```python
from build123d import *

# Parameters (mm, degrees)
F0_W     = 32
F0_H     = 10
F0_R     = 1.6
F1_DEPTH = 3.5
F2_R     = 4.99999
F3_R     = 1


# Not quite as in the source:
# - a fillet or chamfer is up to 0.001 mm smaller than in the source, because OpenCascade refuses the exact size


with BuildPart() as f1:
    # F0 (on Top) → F1 (new body)
    with BuildSketch(Plane.XY):
        with Locations((-9.4221055731, -0.7417218951)):
            Rectangle(F0_W, F0_H)
        with Locations((-20.4221047461, -0.7417218951)):
            Circle(F0_R, mode=Mode.SUBTRACT)
        with Locations((-9.4221055731, -0.7417218951)):
            Circle(F0_R, mode=Mode.SUBTRACT)
        with Locations((1.5778944269, -0.7417218951)):
            Circle(F0_R, mode=Mode.SUBTRACT)
    extrude(amount=F1_DEPTH)

    # F2 (radius 5 in the source; OpenCascade refuses exactly that, so slightly less here)
    f2_edges = [f1.edges().sort_by_distance(p)[0] for p in [
        (6.577894, 4.258278, 1.75),
        (6.577894, -5.741722, 1.75),
        (-25.422106, 4.258278, 1.75),
        (-25.422106, -5.741722, 1.75),
    ]]
    fillet(f2_edges, radius=F2_R)

    # F3
    f3_edges = [f1.edges().sort_by_distance(p)[0] for p in [
        (-9.422106, 4.258278, 3.5),
        (-9.422106, -5.741722, 3.5),
    ]]
    fillet(f3_edges, radius=F3_R)


solid = f1.part
```
CAD build for the part. Positions are in the model's coordinates, mm. Coordinates: 2 decimals unless noted, no trailing zeros. Order: outer loops, then holes, each group sorted by start corner. A loop starts at its lowest first (then second) coordinate and runs counter-clockwise, first axis right, second up. Notation, with made-up numbers: (-28, -9) - (17, -9) arc R13 cw to (17, 0) - close; hole circle Ø1 at (-4, 86). An arc over 180 degrees is marked (long way). Use a Markdown table: item, result. Add a question column.
(1) Saw through at A-A (x = -19.5). Give the cut face in (y, z), then the cut area to 3 significant figures.
(2) Pull direction Y, two halves, no side cores. Call faces 1 (the face through (-9.576, -5.441, 3.215)), 2 (the face through (-11, -1, 2)), 3 (the face through (-10, 1, 3.5)): +Y half, -Y half, draft (parallel to the pull), parting line (faces both ways), or undercut.
(3) Saw through at B-B (z = 1.35). Count the separate pieces of the cut face and the enclosed holes in it, then the cut area to 3 significant figures.
(4) Drill centre lines: line 1 along X through (y, z) = (-2, 0.65); line 2 along X through (y, z) = (-1, 1.9); line 3 along Y through (x, z) = (-8, 2.7). Where is each one in solid material? Low to high. Write a range as [from, to].
Solved:
| question | item | result |
|---|---|---|
| 1 | outline | (-5.74, 0) - (-2.05, 0) - (-2.05, 3.5) - (-4.74, 3.5) arc R1 ccw to (-5.74, 2.5) - close; (0.57, 0) - (4.26, 0) - (4.26, 2.5) arc R1 ccw to (3.26, 3.5) - (0.57, 3.5) - close |
| 1 | area | 25.4 mm² |
| 2 | face 1 | -Y half |
| 2 | face 2 | undercut |
| 2 | face 3 | draft |
| 3 | separate pieces | 1 |
| 3 | enclosed holes | 3 |
| 3 | area | 274 mm² |
| 4 | line 1 | x = [-25.26, -21.41], [-19.43, -10.41], [-8.43, 0.59], [2.57, 6.42] |
| 4 | line 2 | x = [-25.42, -22], [-18.84, -11], [-7.84, 0], [3.16, 6.57] |
| 4 | line 3 | y = [-5.72, -1.47], [-0.01, 4.24] |
